Here's the drawing with two shaded views (mm, measured from the low corner). I have some questions. A direction names the side the tool comes from. Coordinates: 2 decimals unless noted, no trailing zeros. Loops run counter-clockwise (first coordinate to the right, second up) from the corner with the lowest first, then second, coordinate; pieces in that order, holes last. Notation, with made-up numbers: (79.25, -32) -> (98.25, -32) arc R7 ccw to (98.25, -27) -> close; hole circle Ø3 at (6.5, 83). An arc over 180 degrees is marked (long way). Answer as a JSON object with one key per item and string values. Group by question number.
1) I want a section at B-B (x = 12.7). Write out the boundary of the cut face in (y, z) (3 decimals), then the cut area to 3 significant figures.
2) I need wall thicknesses on probe 1 along X at (y, z) = (1.2, 12.7); probe 2 along X at (y, z) = (14, 48); probe 3 along Y at (x, z) = (10.5, 37.5) (3 decimals). Which ranges of each line are inside material? Lowest first, please. Write a range as [from, to].
3) I want a section at D-D (x = 22). Write out the boundary of the cut face in (y, z) (3 decimals).
4) Which directions (+Z, -Z, +X, -X, +Y, -Y) give clear straight access to the entire face, cutting with the end or side of a thin tool? Please do the marked faces 1 and 2.
5) I want a section at C-C (z = 12.7). Write out the boundary of the cut face in (x, y) (3 decimals).
6) I want a section at A-A (y = 38.1). Write out the boundary of the cut face in (x, z) (3 decimals), then the cut area to 3 significant figures.
7) I'm going to push flat-ended pins straight in: pin 1 (8 mm diameter, centred on x = 12.7, z = 34.925, fed in from +Y) (3 decimals); pin 2 (6.5 mm diameter, centred on x = 12.7, y = 50.8, fed in from -Z) (3 decimals); pin 3 (2 mm diameter, centred on x = 23, z = 22.5, fed in from -Y). Where does each tip first touch, or does it pass through?
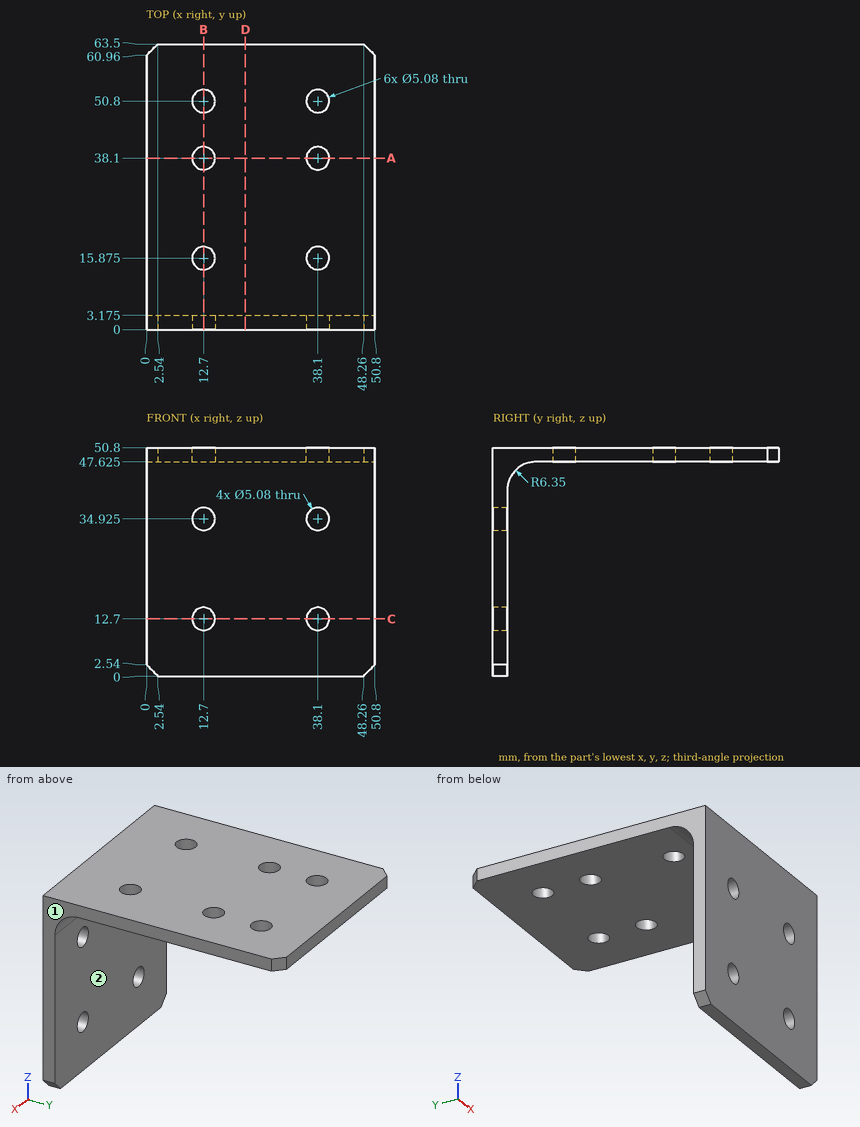
Determined:
{
 "1": {"outline": "(0, 0) -> (3.175, 0) -> (3.175, 10.16) -> (0, 10.16) -> close; (0, 15.24) -> (3.175, 15.24) -> (3.175, 32.385) -> (0, 32.385) -> close; (0, 37.465) -> (3.175, 37.465) -> (3.175, 41.275) arc R6.35 cw to (9.525, 47.625) -> (13.335, 47.625) -> (13.335, 50.8) -> (0, 50.8) -> close; (18.415, 47.625) -> (35.56, 47.625) -> (35.56, 50.8) -> (18.415, 50.8) -> close; (40.64, 47.625) -> (48.26, 47.625) -> (48.26, 50.8) -> (40.64, 50.8) -> close; (53.34, 47.625) -> (63.5, 47.625) -> (63.5, 50.8) -> (53.34, 50.8) -> close", "area": "281 mm^2"},
 "2": {"probe 1": "[0, 10.16], [15.24, 35.56], [40.64, 50.8]", "probe 2": "[0, 10.99], [14.41, 36.39], [39.81, 50.8]", "probe 3": "[0, 3.175]"},
 "3": {"outline": "(0, 0) -> (3.175, 0) -> (3.175, 41.275) arc R6.35 cw to (9.525, 47.625) -> (63.5, 47.625) -> (63.5, 50.8) -> (0, 50.8) -> close"},
 "4": {"face 1": "+Z, -Z, +X, +Y, -Y", "face 2": "-Z, +X, -X, +Y"},
 "5": {"outline": "(0, 0) -> (10.16, 0) -> (10.16, 3.175) -> (0, 3.175) -> close; (15.24, 0) -> (35.56, 0) -> (35.56, 3.175) -> (15.24, 3.175) -> close; (40.64, 0) -> (50.8, 0) -> (50.8, 3.175) -> (40.64, 3.175) -> close"},
 "6": {"outline": "(0, 47.625) -> (10.16, 47.625) -> (10.16, 50.8) -> (0, 50.8) -> close; (15.24, 47.625) -> (35.56, 47.625) -> (35.56, 50.8) -> (15.24, 50.8) -> close; (40.64, 47.625) -> (50.8, 47.625) -> (50.8, 50.8) -> (40.64, 50.8) -> close", "area": "129 mm^2"},
 "7": {"pin 1": "y = 3.175", "pin 2": "z = 47.625", "pin 3": "y = 0"}
}
